from build123d import *

# Parameters (mm, degrees)
F0_W     = 76.2
F0_H     = 76.2
F1_DEPTH = 76.2
F3_DEPTH = 12.7
F4_R     = 12.7
F4_R_2   = 1.279646
F5_DEPTH = 12.7


with BuildPart() as f1:
    # F0 (on Front) → F1 (new body)
    with BuildSketch(Plane.XZ):
        with Locations((-0.882402, 69.589193)):
            Rectangle(F0_W, F0_H)
    extrude(amount=F1_DEPTH)

    # F2 (on face) → F3 (join)
    with BuildSketch(Plane.XZ.offset(76.2)):
        Polygon((0.113132, 71.998739), (-12.586868, 71.998739), (-12.586868, 46.598739), (12.813132, 46.598739), (12.813132, 71.998739), align=None)
    extrude(amount=F3_DEPTH)

    # F4 (on face) → F5 (join)
    with BuildSketch(Plane.YZ.offset(37.217598)):
        with Locations((-41.082326, 71.629331)):
            Circle(F4_R)
        with Locations((-41.082326, 71.629331)):
            Circle(F4_R_2, mode=Mode.SUBTRACT)
    extrude(amount=F5_DEPTH)


solid = f1.part
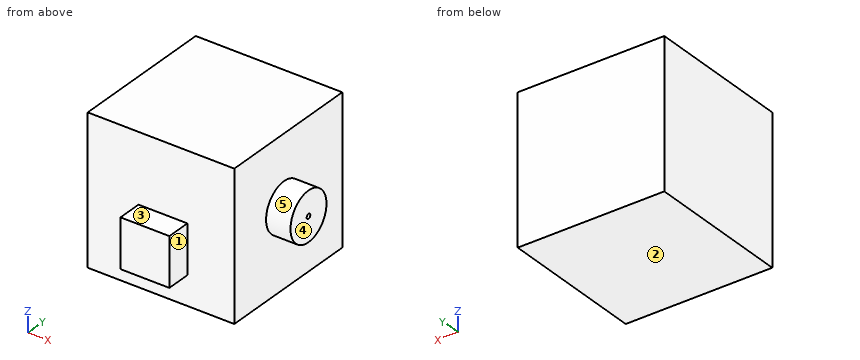
Could you check a few things on this model? Use its own coordinates, in mm. Face numbers are marked on the shaded views. A direction names the side the tool comes from. Give positions to 0.01 mm unless a question says otherwise; leave off trailing zeros. Loops run counter-clockwise (first coordinate to the right, second up) from the corner with the lowest first, then second, coordinate; pieces in that order, holes last. Notation, with made-up numbers: (77, -5) -> (128, -5) arc R18 ccw to (128, 19) -> close; hole circle Ø10 at (69, 2). An arc over 180 degrees is marked (long way). Return JSON: item names as keys, results as strings.
Item 1: If we section it at D-D on z = 61.5: List the corners of the cut face in (x, y) for me, plus the area to 3 significant figures.
Geometry results:
{"outline": "(-38.98, -76.2) -> (-12.59, -76.2) -> (-12.59, -88.9) -> (12.81, -88.9) -> (12.81, -76.2) -> (37.22, -76.2) -> (37.22, -48.74) -> (49.92, -48.74) -> (49.92, -33.42) -> (37.22, -33.42) -> (37.22, 0) -> (-38.98, 0) -> close", "area": "6,320 mm²"}
Item 2: If we section it at A-A on z = 51: List the corners of the cut face in (x, y) for me, plus the area to 3 significant figures.
Geometry results:
{"outline": "(-38.98, -76.2) -> (-12.59, -76.2) -> (-12.59, -88.9) -> (12.81, -88.9) -> (12.81, -76.2) -> (37.22, -76.2) -> (37.22, 0) -> (-38.98, 0) -> close", "area": "6,130 mm²"}
Item 3: I need wall thicknesses on L1, parallel to Y at x = -14, z = 48; L2, parallel to X at y = -13, z = 83; L3, parallel to Z at x = 37.5, y = -32. Which ranges of each line are inside material? Lowest first, please. Write a range as from..to.
Geometry results:
{"L1": "y = -76.2..0", "L2": "x = -38.98..37.22", "L3": "z = 62.75..80.51"}
Item 4: If we section it at B-B on y = -30: List the corners of the cut face in (x, z) for me.
Geometry results:
{"outline": "(-38.98, 31.49) -> (37.22, 31.49) -> (37.22, 65.43) -> (49.92, 65.43) -> (49.92, 77.83) -> (37.22, 77.83) -> (37.22, 107.69) -> (-38.98, 107.69) -> close"}
Item 5: Which directions (+Z, -Z, +X, -X, +Y, -Y) give clear straight access to the entire face, cutting with the end or side of a thin tool? Please do the marked faces 1, 2, 3, 4 and 5.
Geometry results:
{"face 1": "+Z, -Z, +X, -Y", "face 2": "-Z, +X, -X, +Y, -Y", "face 3": "+Z, +X, -X, -Y", "face 4": "+Z, -Z, +X, +Y, -Y", "face 5": "+X"}
Item 6: I'm going to push flat-ended pins straight in: pin 1 (4 mm diameter, centred on x = -15, z = 83.5, fed in from -Y); pin 2 (1.5 mm diameter, centred on y = -41.08, z = 71.63, fed in from +X); pin 3 (4 mm diameter, centred on y = -82, z = 65.5, fed in from +X). Where does each tip first touch, or does it pass through?
Geometry results:
{"pin 1": "stops at y = -76.2", "pin 2": "stops at x = 37.22", "pin 3": "stops at x = 12.81"}
Item 7: If we section it at C-C on x = 36: List the corners of the cut face in (y, z) for me, plus the area to 3 significant figures.
Geometry results:
{"outline": "(-76.2, 31.49) -> (0, 31.49) -> (0, 107.69) -> (-76.2, 107.69) -> close", "area": "5,810 mm²"}
